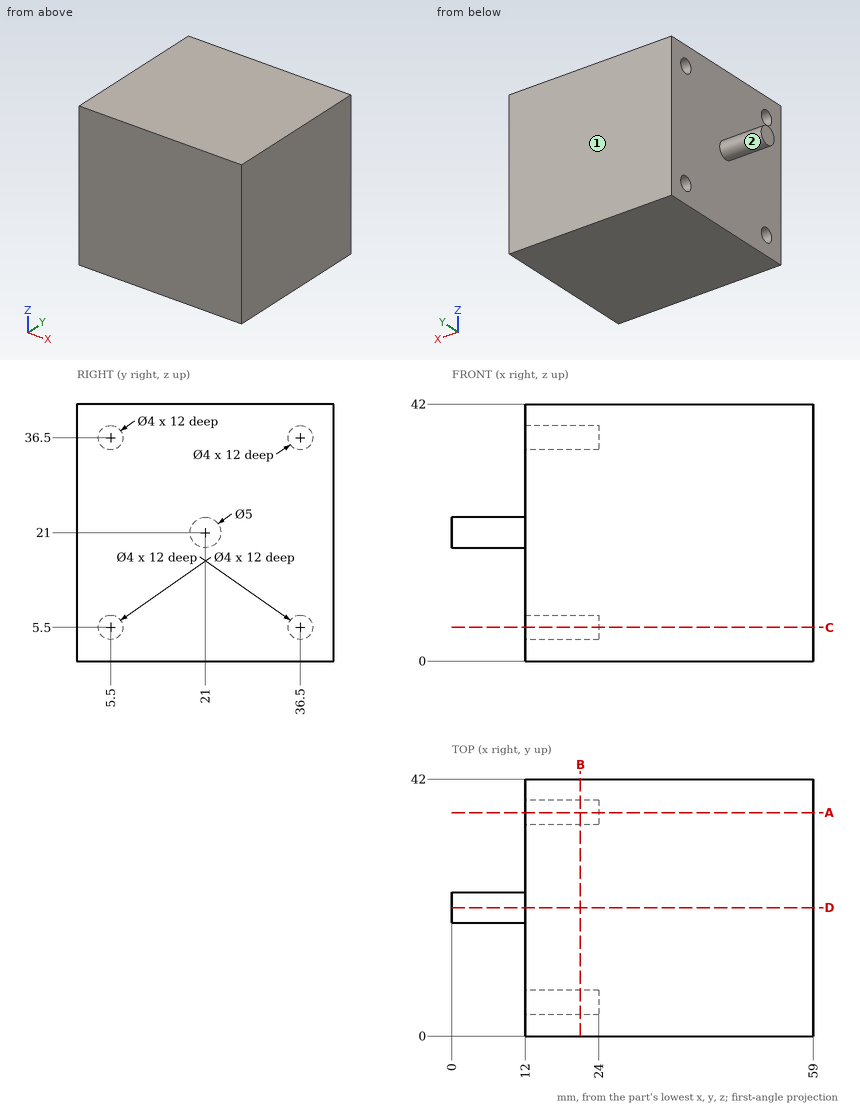
Study the drawing (mm; zero at the part's minimum x, y, z) and answer. A direction names the side the tool comes from. Coordinates: 2 decimals unless noted, no trailing zeros. Write each loop counter-clockwise with the first axis right and the second up, starting at its lowest first coordinate (ties: lowest second). Pieces come first, ordered by that corner, then holes. Notation, with made-up numbers: M -5.5,-15.5 L 31.5,-15.5 A20 ccw 31.5,-10.5 Z; hole C -16.5,58 d8. An arc over 180 degrees is marked long. Use a Markdown table: item, result. Add a question column.
1. Section B-B (x = 21) is taken. Give the vertices of the cut face in (y, z), plus the area to 3 significant figures.
2. Which of the six approach directions +Z, -Z, +X, -X, +Y, -Y give full straight-line access (tool end or side, diameter ignored) to the marked faces 1 and 2?
3. Straight lines are drawn through the part: line 1 along Y through (x, z) = (18, 5.5); line 2 along Y through (x, z) = (20, 5). For each, find the intervals that lie inside material, in ascending order. Write a range as [from, to].
4. Given P1, Ø1.2, axis at y = 36.5, z = 5, coming from the -X side; P2, Ø1.5, axis at y = 10, z = 15, coming from the -X side, each flat-ended and moving along its own axis, determine where each tip first touches the part or whether it passes through.
5. Section D-D (y = 21) is taken. Give the vertices of the cut face in (x, z).
6. Section A-A (y = 36.5) is taken. Give the vertices of the cut face in (x, z), plus the area to 3 significant figures.
Data:
| question | item | result |
|---|---|---|
| 1 | outline | M 0,0 L 42,0 L 42,42 L 0,42 Z; hole C 5.5,5.5 d4; hole C 5.5,36.5 d4; hole C 36.5,5.5 d4; hole C 36.5,36.5 d4 |
| 1 | area | 1,710 mm2 |
| 2 | face 1 | +Z, -Z, +X, -X, +Y |
| 2 | face 2 | -X |
| 3 | line 1 | y = [0, 3.5], [7.5, 34.5], [38.5, 42] |
| 3 | line 2 | y = [0, 3.56], [7.44, 34.56], [38.44, 42] |
| 4 | P1 | stops at x = 24 |
| 4 | P2 | stops at x = 12 |
| 5 | outline | M 0,18.5 L 12,18.5 L 12,0 L 59,0 L 59,42 L 12,42 L 12,23.5 L 0,23.5 Z |
| 6 | outline | M 12,0 L 59,0 L 59,42 L 12,42 L 12,38.5 L 24,38.5 L 24,34.5 L 12,34.5 L 12,7.5 L 24,7.5 L 24,3.5 L 12,3.5 Z |
| 6 | area | 1,880 mm2 |
